Source: CAD feature listing. Evaluate the final solid. Frame: model axes, mm. A direction names the side the tool comes from. Round coordinates to 2 decimals unless told otherwise and drop trailing zeros. Write each loop counter-clockwise with the first axis right and the second up, starting at its lowest first coordinate (ties: lowest second). Pieces come first, ordered by that corner, then holes. Notation, with made-up numbers: M 51,-6 L 106,-6 A34 cw 106,26 Z; hole C -36,51.25 d1. An arc over 180 degrees is marked long. Use a Markdown table: item, result.
```python
from build123d import *

# Parameters (mm, degrees)
CUT_EXTRUDE1_DEPTH      = 78.575769413
CUT_EXTRUDE1_DEPTH_BACK = 9
SKETCH2_W               = 40
SKETCH2_H               = 94
SKETCH3_W               = 10
SKETCH3_H               = 40
CUT_EXTRUDE2_DEPTH      = 78.05193054
SKETCH4_R               = 1.5
BOSS_EXTRUDE1_DEPTH     = 4
MOVE_START              = -46.130250379
MOVE_FACE1_OUTLINE_W    = 16.928932188
MOVE_FACE1_OUTLINE_H    = 4
MOVE_FACE1_DEPTH        = 0.963891216
MOVE_START_2            = 45.166359163
MOVE_FACE1_2_OUTLINE_W  = 16.928932188
MOVE_FACE1_2_OUTLINE_H  = 4
MOVE_FACE1_2_DEPTH      = 0.963891216
MOVE_START_3            = -28.692666648
MOVE_FACE1_3_DEPTH      = 1.57682047
MOVE_START_4            = 27.115846178
MOVE_FACE1_4_DEPTH      = 1.57682047
FILLET1_R               = 2


with BuildPart() as part:
    # Sketch1 → Revolve1 (revolve)
    with BuildSketch(Plane.XY, mode=Mode.PRIVATE) as revolve1_sk:
        Polygon((0, 47), (23.071067812, 47), (40, 30.071067812), (40, 0), (35, 0), (35, 28), (20, 43), (0, 43), align=None)
    revolve(revolve1_sk.sketch.rotate(Axis((0, 0, 0), (1, 0, 0)), 90), axis=Axis((0, 0, 0), (1, 0, 0)))

    # Sketch2 → Cut-Extrude1 (cut, two sides: drawn at the far end of the back side and taken through both)
    with BuildSketch(Plane.XY.offset(-CUT_EXTRUDE1_DEPTH_BACK)):
        with Locations((20, 0)):
            Rectangle(SKETCH2_W, SKETCH2_H)
    extrude(amount=CUT_EXTRUDE1_DEPTH + CUT_EXTRUDE1_DEPTH_BACK, mode=Mode.SUBTRACT)

    # Sketch3 → Cut-Extrude2 (cut, through all)
    with BuildSketch(Plane(origin=(40, 0, 0), x_dir=(0, 0, -1), z_dir=(1, 0, 0))):
        with Locations((14, 0)):
            Rectangle(SKETCH3_W, SKETCH3_H)
    extrude(amount=-CUT_EXTRUDE2_DEPTH, mode=Mode.SUBTRACT)

    # Sketch4 → Boss-Extrude1 (add)
    # profile 1 of 2: a face of its own
    with BuildSketch(Plane.XY.offset(-9)):
        with BuildLine():
            Line((23.071067812, 46.130250379), (38, 46.130250379))
            ThreePointArc((38, 46.130250379), (39.414213562, 45.544463941), (40, 44.130250379))
            Line((40, 44.130250379), (40, 28.692666648))
            Line((40, 28.692666648), (32.929135877, 28.692666648))
            Line((32.929135877, 28.692666648), (23.071067812, 38.901502546))
            Line((23.071067812, 38.901502546), (23.071067812, 46.130250379))
        make_face()
        with Locations((36, 42.130250379)):
            Circle(SKETCH4_R, mode=Mode.SUBTRACT)
    # profile 2 of 2: a face of its own
    with BuildSketch(Plane.XY.offset(-9)):
        with BuildLine():
            Line((23.071067812, -38.901502546), (23.071067812, -46.130250379))
            Line((23.071067812, -46.130250379), (38, -46.130250379))
            ThreePointArc((38, -46.130250379), (39.414213562, -45.544463941), (40, -44.130250379))
            Line((40, -44.130250379), (40, -28.692666648))
            Line((40, -28.692666648), (32.929135877, -28.692666648))
            Line((32.929135877, -28.692666648), (23.071067812, -38.901502546))
        make_face()
        with Locations(Location((36, -42.130250379, 0), (0, 0, 180))):
            Circle(SKETCH4_R, mode=Mode.SUBTRACT)
    extrude(amount=-BOSS_EXTRUDE1_DEPTH)


with BuildPart() as move_face1_tool:
    # Move Face1: read off the stored shape, not the designer's step
    # Move Face1 outline → Move Face1 (new body)
    with BuildSketch(Plane(origin=(0, 0, 0), x_dir=(1, 0, 0), z_dir=(0, 1, 0)).offset(MOVE_START)):
        with Locations((29.535533906, 11)):
            Rectangle(MOVE_FACE1_OUTLINE_W, MOVE_FACE1_OUTLINE_H)
    extrude(amount=MOVE_FACE1_DEPTH)


with BuildPart() as part_1:
    add(part.part)


with BuildPart() as part_2:
    # Move Face1: joined with move_face1_tool
    add(part_1.part.fuse(move_face1_tool.part, tol=0.00001))


with BuildPart() as move_face1_2_tool:
    # Move Face1 2 outline → Move Face1 2 (new body)
    with BuildSketch(Plane(origin=(0, 0, 0), x_dir=(1, 0, 0), z_dir=(0, 1, 0)).offset(MOVE_START_2)):
        with Locations((29.535533906, 11)):
            Rectangle(MOVE_FACE1_2_OUTLINE_W, MOVE_FACE1_2_OUTLINE_H)
    extrude(amount=MOVE_FACE1_2_DEPTH)


with BuildPart() as part_3:
    add(part_2.part)


with BuildPart() as part_4:
    # Move Face1 2: joined with move_face1_2_tool
    add(part_3.part.fuse(move_face1_2_tool.part, tol=0.00001))


with BuildPart() as move_face1_3_tool:
    # Move Face1 3 outline → Move Face1 3 (new body)
    with BuildSketch(Plane(origin=(0, 0, 0), x_dir=(1, 0, 0), z_dir=(0, 1, 0)).offset(MOVE_START_3)):
        with BuildLine():
            Line((40, 13), (38.57076781, 13.000001435))
            add(Edge.make_bspline(
                [(38.57076781, 13.000001435), (38.71437599, 12.652027053), (38.853897492, 12.302357037), (39.340707465, 11.036237384), (39.662536412, 10.10974197), (39.965458557, 9.114909953), (39.982798274, 9.057475387), (40.00000015, 9.000000045)],
                knots=[15.019424216, 15.019424216, 15.019424216, 15.019424216, 16.148697383, 16.148697383, 19.088168409, 19.088168409, 19.268134003, 19.268134003, 19.268134003, 19.268134003], degree=3))
            Line((40.00000015, 9.000000045), (40, 13))
        make_face()
    extrude(amount=MOVE_FACE1_3_DEPTH)


with BuildPart() as part_5:
    add(part_4.part)


with BuildPart() as part_6:
    # Move Face1 3: joined with move_face1_3_tool
    add(part_5.part.fuse(move_face1_3_tool.part, tol=0.00001))


with BuildPart() as move_face1_4_tool:
    # Move Face1 4 outline → Move Face1 4 (new body)
    with BuildSketch(Plane(origin=(0, 0, 0), x_dir=(1, 0, 0), z_dir=(0, 1, 0)).offset(MOVE_START_4)):
        with BuildLine():
            Line((40, 13), (38.57076781, 13.000001435))
            add(Edge.make_bspline(
                [(38.57076781, 13.000001435), (38.71437599, 12.652027053), (38.853897492, 12.302357037), (39.340707465, 11.036237384), (39.662536412, 10.10974197), (39.965458557, 9.114909953), (39.982798274, 9.057475387), (40.00000015, 9.000000045)],
                knots=[15.019424216, 15.019424216, 15.019424216, 15.019424216, 16.148697383, 16.148697383, 19.088168409, 19.088168409, 19.268134003, 19.268134003, 19.268134003, 19.268134003], degree=3))
            Line((40.00000015, 9.000000045), (40, 13))
        make_face()
    extrude(amount=MOVE_FACE1_4_DEPTH)


with BuildPart() as part_7:
    add(part_6.part)


with BuildPart() as part_8:
    # Move Face1 4: joined with move_face1_4_tool
    add(part_7.part.fuse(move_face1_4_tool.part, tol=0.00001))

    # Fillet1
    fillet1_edges = [part_8.edges().sort_by_distance(p)[0] for p in [
        (37.5, -20, -9),
        (37.5, 20, -9),
    ]]
    fillet(fillet1_edges, radius=FILLET1_R)


solid = part_8.part
```
Q1. Section A-A on x = 36. Return loops of the section in (y, z).
Results are:
| item | result |
|---|---|
| outline | M -46.13,-13 L -43.63,-13 L -43.63,-9 L -46.13,-9 Z; M -40.63,-13 L -31.49,-13 A34.07 ccw 31.49,-13 L 40.63,-13 L 40.63,-9 L 22,-9 A2 ccw 20,-11 L 20,-19 L -20,-19 L -20,-11 A2 ccw -22,-9 L -40.63,-9 Z; M 43.63,-13 L 46.13,-13 L 46.13,-9 L 43.63,-9 Z |
Q2. Reachability of faces 1 (the flat face through (38, 20, -15)), 2 (the flat face through (35, 0, -20)), 3 (the flat face through (29, 46.13, -11)) from +Z, -Z, +X, -X, +Y, -Y: full face, straight path, thin tool, end or side. Return the list, or none.
Results are:
| item | result |
|---|---|
| face 1 | +Z, +X, -X |
| face 2 | +Z, -X |
| face 3 | +Z, -Z, +X, -X, +Y |
Q3. Line query: L1, parallel to Y at x = 36, z = -11; L2, parallel to Y at x = 36, z = -10; L3, parallel to X at y = 17.5, z = -21.5. Output: solid intervals per line, ascending.
Results are:
| item | result |
|---|---|
| L1 | -46.13 to -43.63, -40.63 to -20, 20 to 40.63, 43.63 to 46.13 |
| L2 | -46.13 to -43.63, -40.63 to -20.27, 20.27 to 40.63, 43.63 to 46.13 |
| L3 | 35 to 40 |
Q4. Section C-C on x = 9.5. Return loops of the section in (y, z), plus the area to 3 significant figures.
Results are:
| item | result |
|---|---|
| outline | M -46.13,-9 A47 ccw 46.13,-9 L 42.05,-9 A43 cw -42.05,-9 Z |
| area | 493 mm^2 |
Q5. Mould query, pull axis Y, two halves, no side actions, for faces 4 (the conical face through (35.416, -0.626, -34.649)), 5 (the cylindrical face through (39.4, -45.56, -10.97)), 6 (the flat face through (38, 0, -19)). Classes: +Y half, -Y half, draft (parallel to the pull), parting line (faces both ways), or undercut.
Results are:
| item | result |
|---|---|
| face 4 | parting line |
| face 5 | -Y half |
| face 6 | undercut |
Q6. First-contact query: pin 1 Ø0.8 at (y, z) = (-45.5, -11.5) entering from -X; pin 2 Ø19 at (x, y) = (31.5, -41.5) entering from -Z; pin 3 Ø4 at (x, y) = (36, 42.13) entering from -Z; pin 4 Ø4 at (y, z) = (-5.5, -19.5) entering from -X. Flat tips, straight axial feed; report the tip coordinate or a pass-through.
Results are:
| item | result |
|---|---|
| pin 1 | x = 0 |
| pin 2 | z = -29.16 |
| pin 3 | z = -13 |
| pin 4 | x = 35 |
